from build123d import *

# Parameters (mm, degrees)
F1_DEPTH      = 10
F1_DEPTH_BACK = 10
F2_R          = 8
F3_DEPTH      = 10
F3_DEPTH_BACK = 10


with BuildPart() as f1:
    # F0 (on Front) → F1 (new body, two sides)
    with BuildSketch(Plane.XZ) as f1_sk:
        with BuildLine():
            Line((50, 36), (-125, 36))
            Line((-125, 36), (-125, 0))
            ThreePointArc((-125, 0), (-112.5, -12.5), (-100, 0))
            Line((-100, 0), (-100, 16))
            Line((-100, 16), (25, 16))
            Line((25, 16), (25, 0))
            ThreePointArc((25, 0), (37.5, -12.5), (50, 0))
            Line((50, 0), (50, 36))
        make_face()
    extrude(amount=F1_DEPTH)
    extrude(f1_sk.sketch, amount=-F1_DEPTH_BACK)

    # F2 (on Front) → F3 (cut, two sides)
    with BuildSketch(Plane.XZ) as f3_sk:
        with Locations((-112.5, 0)):
            Circle(F2_R)
        with Locations((37.5, 0)):
            Circle(F2_R)
    extrude(amount=F3_DEPTH, mode=Mode.SUBTRACT)
    extrude(f3_sk.sketch, amount=-F3_DEPTH_BACK, mode=Mode.SUBTRACT)


solid = f1.part
Design review of the part built by this model. Coordinates are the model's own, in mm. A direction names the side the tool comes from. Give positions to 0.01 mm unless a question says otherwise; leave off trailing zeros. Loops run counter-clockwise (first coordinate to the right, second up) from the corner with the lowest first, then second, coordinate; pieces in that order, holes last. Notation, with made-up numbers: M 32.25,21 L 90.25,21 A12 ccw 90.25,43 Z; hole C -36,46.25 d7. An arc over 180 degrees is marked long. Answer as a JSON object with one key per item and string values.
Item 1: Wall thickness on line 1 along Z through (x, y) = (37.5, -5); line 2 along X through (y, z) = (-4.5, 13); line 3 along X through (y, z) = (5.75, 2.5): over which ranges is each line inside the solid? List them lowest first.
Output values:
{"line 1": "z = -12.5 to -8, 8 to 36", "line 2": "x = -125 to -100, 25 to 50", "line 3": "x = -125 to -120.1, -104.9 to -100, 25 to 29.9, 45.1 to 50"}
Item 2: We need section C-C (x = -84.5). State the section outline as (y, z) points, and give its area (3 significant figures).
Output values:
{"outline": "M -10,16 L 10,16 L 10,36 L -10,36 Z", "area": "400 mm2"}
Item 3: Machinability: for faces 1 (the face through (-39, -10, 23)), 2 (the face through (-100, 0, 8)), which of the approach directions +Z, -Z, +X, -X, +Y, -Y give a long, thin tool a straight path to every point of the face, cutting with its end or side? Answer none if there is none.
Output values:
{"face 1": "+Z, -Z, +X, -X, -Y", "face 2": "-Z, +Y, -Y"}
Item 4: We need section B-B (x = -112.5). State the section outline as (y, z) points.
Output values:
{"outline": "M -10,-12.5 L 10,-12.5 L 10,-8 L -10,-8 Z; M -10,8 L 10,8 L 10,36 L -10,36 Z"}
Item 5: For P1, Ø6, axis at x = -66, y = -2, coming from the -Z side; P2, Ø5, axis at x = 30, y = -7, coming from the -Z side; P3, Ø9.5, axis at x = 37.5, z = 0, coming from the +Y side, all flat-tipped, find the tip position at first contact; note any pin that passes through.
Output values:
{"P1": "stops at z = 16", "P2": "stops at z = -11.46", "P3": "passes through"}
Item 6: We need section A-A (y = 2). State the section outline as (x, z) points, and give its area (3 significant figures).
Output values:
{"outline": "M -125,0 A12.5 ccw -100,0 L -100,16 L 25,16 L 25,0 A12.5 ccw 50,0 L 50,36 L -125,36 Z; hole C -112.5,0 d16; hole C 37.5,0 d16", "area": "4,390 mm2"}
